Here's how the part is built. I have some questions about the finished solid (model axes, mm). Face numbers are marked on the shaded views. A direction names the side the tool comes from. Round coordinates to 2 decimals unless told otherwise and drop trailing zeros. Order: outer loops, then holes, each group sorted by start corner. A loop starts at its lowest first (then second) coordinate and runs counter-clockwise, first axis right, second up. Notation, with made-up numbers: (-31.75, 32.25) -> (-17.75, 32.25) arc R27 cw to (-17.75, 68.25) -> close; hole circle Ø1 at (28, 36.5). An arc over 180 degrees is marked (long way). Answer in a Markdown table with one row per item.
```python
from build123d import *

# Parameters (mm, degrees)
BOSS_EXTRUDE1_DEPTH     = 17.5
CUT_EXTRUDE2_DEPTH      = 63.681735777
CUT_EXTRUDE2_DEPTH_BACK = 14
CUT_EXTRUDE3_DEPTH      = 55.16871791
CUT_EXTRUDE3_DEPTH_BACK = 55.16871791
SKETCH4_R               = 2
CUT_EXTRUDE5_DEPTH      = 55.16871791
CUT_EXTRUDE5_DEPTH_BACK = 55.16871791
SKETCH6_R               = 2


with BuildPart() as part:
    # Sketch1 → Boss-Extrude1 (new, symmetric)
    with BuildSketch(Plane(origin=(0, 0, 0), x_dir=(0, 0, -1), z_dir=(1, 0, 0))):
        with BuildLine():
            Line((0, 0), (11, 0))
            ThreePointArc((11, 0), (11.707106781, 0.292893219), (12, 1))
            Line((12, 1), (12, 17))
            ThreePointArc((12, 17), (12.292893219, 17.707106781), (13, 18))
            Line((13, 18), (35, 18))
            ThreePointArc((35, 18), (35.707106781, 17.707106781), (36, 17))
            Line((36, 17), (36, 1))
            ThreePointArc((36, 1), (36.292893219, 0.292893219), (37, 0))
            Line((37, 0), (48, 0))
            Line((48, 0), (48, 2))
            Line((48, 2), (39, 2))
            ThreePointArc((39, 2), (38.292893219, 2.292893219), (38, 3))
            Line((38, 3), (38, 17))
            ThreePointArc((38, 17), (37.121320344, 19.121320344), (35, 20))
            Line((35, 20), (13, 20))
            ThreePointArc((13, 20), (10.878679656, 19.121320344), (10, 17))
            Line((10, 17), (10, 3))
            ThreePointArc((10, 3), (9.707106781, 2.292893219), (9, 2))
            Line((9, 2), (0, 2))
            Line((0, 2), (0, 0))
        make_face()
    extrude(amount=BOSS_EXTRUDE1_DEPTH, both=True)

    # Sketch3 → Cut-Extrude2 (cut, two sides: drawn at the far end of the back side and taken through both)
    with BuildSketch(Plane(origin=(17.5, 0, 0), x_dir=(0, 0, -1), z_dir=(1, 0, 0)).offset(-CUT_EXTRUDE2_DEPTH_BACK)):
        with BuildLine():
            Line((10, 17), (10, 16))
            Line((10, 16), (12, 16))
            Line((12, 16), (12, 17))
            ThreePointArc((12, 17), (12.292893219, 17.707106781), (13, 18))
            Line((13, 18), (35, 18))
            ThreePointArc((35, 18), (35.707106781, 17.707106781), (36, 17))
            Line((36, 17), (36, 16))
            Line((36, 16), (38, 16))
            Line((38, 16), (38, 17))
            ThreePointArc((38, 17), (37.121320344, 19.121320344), (35, 20))
            Line((35, 20), (13, 20))
            ThreePointArc((13, 20), (10.878679656, 19.121320344), (10, 17))
        make_face()
    extrude(amount=CUT_EXTRUDE2_DEPTH + CUT_EXTRUDE2_DEPTH_BACK, mode=Mode.SUBTRACT)

    # Sketch4 → Cut-Extrude3 (cut, two sides: drawn at the far end of the back side and taken through both)
    with BuildSketch(Plane(origin=(0, 2, 0), x_dir=(1, 0, 0), z_dir=(0, 1, 0)).offset(-CUT_EXTRUDE3_DEPTH_BACK)):
        with Locations(Location((-12.5, 43, 0), (0, 0, 270))):
            Circle(SKETCH4_R)
        with Locations(Location((12.5, 43, 0), (0, 0, 270))):
            Circle(SKETCH4_R)
    extrude(amount=CUT_EXTRUDE3_DEPTH + CUT_EXTRUDE3_DEPTH_BACK, mode=Mode.SUBTRACT)

    # Sketch6 → Cut-Extrude5 (cut, two sides: drawn at the far end of the back side and taken through both)
    with BuildSketch(Plane(origin=(0, 2, 0), x_dir=(1, 0, 0), z_dir=(0, 1, 0)).offset(-CUT_EXTRUDE5_DEPTH_BACK)):
        with Locations(Location((-12.5, 5, 0), (0, 0, 90))):
            Circle(SKETCH6_R)
        with Locations(Location((12.5, 5, 0), (0, 0, 90))):
            Circle(SKETCH6_R)
        with Locations(Location((-9.5, 24, 0), (0, 0, 270))):
            Circle(SKETCH6_R)
        with Locations(Location((-1.5, 24, 0), (0, 0, 270))):
            Circle(SKETCH6_R)
    extrude(amount=CUT_EXTRUDE5_DEPTH + CUT_EXTRUDE5_DEPTH_BACK, mode=Mode.SUBTRACT)


solid = part.part
```
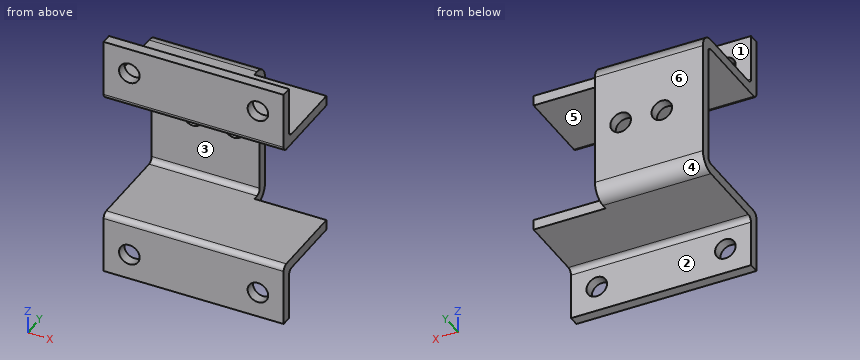
1. We'd pull the mould along Z, two halves only. Please class the marked faces 4, 5 and 6: released by +Z, released by -Z, zero draft, split by the parting line, or undercut.
Numbers:
| item | result |
|---|---|
| face 4 | released by -Z |
| face 5 | undercut |
| face 6 | zero draft |
2. Suppose I cut it at A-A on x = 8. Write out the boundary of the cut face in (y, z), then the cut area to 3 significant figures.
Numbers:
| item | result |
|---|---|
| outline | (0, -48) -> (2, -48) -> (2, -39) arc R1 cw to (3, -38) -> (16, -38) -> (16, -36) -> (1, -36) arc R1 ccw to (0, -37) -> close; (0, -11) arc R1 ccw to (1, -12) -> (16, -12) -> (16, -10) -> (3, -10) arc R1 cw to (2, -9) -> (2, 0) -> (0, 0) -> close |
| area | 104 mm2 |
3. For the marked faces 1, 2 and 3, which set-ups out of +Z, -Z, +X, -X, +Y, -Y let a thin tool reach every point of the face, with its end or its side?
Numbers:
| item | result |
|---|---|
| face 1 | +Z, +X, -X, +Y |
| face 2 | -Z, +X, -X, +Y |
| face 3 | +X, -X, -Y |
4. For pin 1 Ø8 at (x, y) = (-0.5, 11) entering from +Z; pin 2 Ø3 at (x, z) = (-12.5, -5) entering from +Y; pin 3 Ø5 at (x, z) = (-1.5, -24) entering from -Y; pin 4 Ø7 at (x, y) = (4, 9.5) entering from -Z, each with a flat end and sliding along its axis, tell me the tip position at first contact or that it passes through.
Numbers:
| item | result |
|---|---|
| pin 1 | stops at z = -10 |
| pin 2 | passes through |
| pin 3 | stops at y = 18 |
| pin 4 | stops at z = -38 |
5. Please list where these lines run through material, in increasing order: line 1 along X through (y, z) = (19.3, -24); line 2 along X through (y, z) = (1.2, -43); line 3 along Z through (x, y) = (10, 8.75).
Numbers:
| item | result |
|---|---|
| line 1 | x = -17.5 to -11.5, -7.5 to -3.5, 0.5 to 3.5 |
| line 2 | x = -17.5 to -14.5, -10.5 to 10.5, 14.5 to 17.5 |
| line 3 | z = -38 to -36, -12 to -10 |
6. Suppose I cut it at B-B on z = -24. Write out the boundary of the cut face in (x, y).
Numbers:
| item | result |
|---|---|
| outline | (-17.5, 18) -> (-11.5, 18) -> (-11.5, 20) -> (-17.5, 20) -> close; (-7.5, 18) -> (-3.5, 18) -> (-3.5, 20) -> (-7.5, 20) -> close; (0.5, 18) -> (3.5, 18) -> (3.5, 20) -> (0.5, 20) -> close |
7. Suppose I cut it at C-C on y = 7.5. Write out the boundary of the cut face in (x, z).
Numbers:
| item | result |
|---|---|
| outline | (-17.5, -38) -> (17.5, -38) -> (17.5, -36) -> (-17.5, -36) -> close; (-17.5, -12) -> (17.5, -12) -> (17.5, -10) -> (-17.5, -10) -> close |
8. Suppose I cut it at D-D on x = 12.5. Write out the boundary of the cut face in (y, z), then the cut area to 3 significant figures.
Numbers:
| item | result |
|---|---|
| outline | (0, -48) -> (2, -48) -> (2, -45) -> (0, -45) -> close; (0, -41) -> (2, -41) -> (2, -39) arc R1 cw to (3, -38) -> (16, -38) -> (16, -36) -> (1, -36) arc R1 ccw to (0, -37) -> close; (0, -11) arc R1 ccw to (1, -12) -> (16, -12) -> (16, -10) -> (3, -10) arc R1 cw to (2, -9) -> (2, -7) -> (0, -7) -> close; (0, -3) -> (2, -3) -> (2, 0) -> (0, 0) -> close |
| area | 88.0 mm2 |
